from build123d import *

# Parameters (mm, degrees)
F1_DEPTH = 9.525
F2_DEPTH = 9.525
F3_D     = 12.7


with BuildPart() as f1:
    # F0 (on Right) → F1 (new body)
    with BuildSketch(Plane.YZ):
        Polygon((0, 57.15), (0, 0), (225.425, 0), (225.425, 37.3376765309), (225.425, 57.15), (156.083, 57.15), align=None)
    extrude(amount=F1_DEPTH)

    # F0 (on Right) → F2 (join)
    with BuildSketch(Plane.YZ):
        Polygon((0, 57.15), (0, 0), (225.425, 0), (225.425, 37.3376765309), (225.425, 57.15), (156.083, 57.15), align=None)
        with BuildLine():
            Line((225.425, 57.15), (225.425, 37.3376765309))
            Line((225.425, 37.3376765309), (319.5570650431, 64.2329913682))
            ThreePointArc((319.5570650431, 64.2329913682), (305.0721225399, 65.8972639905), (296.0065399278, 77.3164835165))
            Line((296.0065399278, 77.3164835165), (225.425, 57.15))
        make_face()
        with BuildLine():
            Line((309.0900320761, 100.8670086318), (156.083, 57.15))
            Line((156.083, 57.15), (225.425, 57.15))
            Line((225.425, 57.15), (296.0065399278, 77.3164835165))
            ThreePointArc((296.0065399278, 77.3164835165), (297.67081255, 91.8014260196), (309.0900320761, 100.8670086318))
        make_face()
        with BuildLine():
            Line((314.3235485596, 82.55), (319.5570650431, 64.2329913682))
            ThreePointArc((319.5570650431, 64.2329913682), (329.5321150438, 71.0782082701), (333.3735485596, 82.55))
            ThreePointArc((333.3735485596, 82.55), (325.7953402895, 97.7585664842), (309.0900320761, 100.8670086318))
            Line((309.0900320761, 100.8670086318), (314.3235485596, 82.55))
        make_face()
        with BuildLine():
            ThreePointArc((296.0065399278, 77.3164835165), (305.0721225399, 65.8972639905), (319.5570650431, 64.2329913682))
            Line((319.5570650431, 64.2329913682), (314.3235485596, 82.55))
            Line((314.3235485596, 82.55), (296.0065399278, 77.3164835165))
        make_face()
        with BuildLine():
            Line((314.3235485596, 82.55), (309.0900320761, 100.8670086318))
            ThreePointArc((309.0900320761, 100.8670086318), (297.67081255, 91.8014260196), (296.0065399278, 77.3164835165))
            Line((296.0065399278, 77.3164835165), (314.3235485596, 82.55))
        make_face()
    extrude(amount=F2_DEPTH)

    # F3 (through all)
    with Locations(Plane(origin=(0, 0, 0), x_dir=(0, 1, 0), z_dir=(-1, 0, 0))):
        with Locations((314.3235485596, -82.55)):
            Hole(F3_D / 2)


solid = f1.part
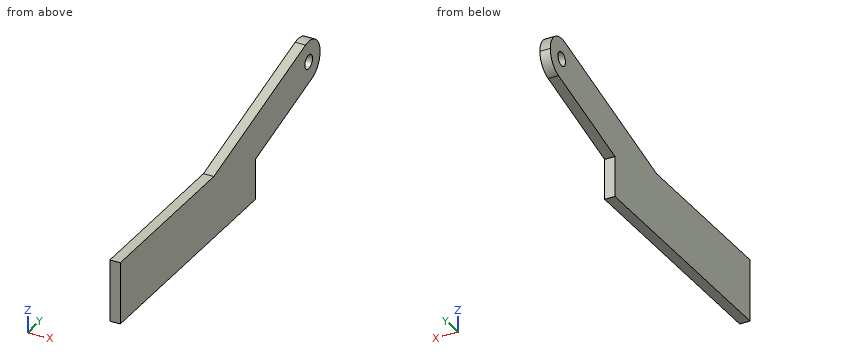
Part model, mm, in its own coordinate system. Give positions to 0.01 mm unless a question says otherwise; leave off trailing zeros. Loops run counter-clockwise (first coordinate to the right, second up) from the corner with the lowest first, then second, coordinate; pieces in that order, holes last. Notation, with made-up numbers: M 3.25,31 L 43.25,31 A30 cw 43.25,60 Z; hole C -10,8.25 d3. An arc over 180 degrees is marked long. Put each result on its own line as item: value. Start each with the question number.
1) Saw through at A-A (x = 6.5). List the corners of the cut face in (y, z) (3 decimals), then the cut area to 3 significant figures.
2) Saw through at C-C (y = 265.5). List the corners of the cut face in (x, z) (3 decimals), then the cut area to 3 significant figures.
3) Flat gauge pins, fed straight in: pin 1 (3 mm diameter, centred on x = 4, y = 82, fed in from +Z); pin 2 (5 mm diameter, centred on x = 7, z = 18, fed in from +Y) (3 decimals); pin 3 (4 mm diameter, centred on x = 7, y = 292, fed in from +Z); pin 4 (11.5 mm diameter, centred on y = 314.32, z = 82.55, fed in from +X). Where does each tip first touch, or does it go through?
4) Probe probe 1 along Z at (x, y) = (3, 150.5); probe 2 along Y at (x, z) = (3.5, 25) (3 decimals); probe 3 along Z at (x, y) = (4, 282). List the from-to ranges inside material, lowest first.
5) Saw through at B-B (y = 128). List the corners of the cut face in (x, z) (3 decimals).
Numbers:
1. outline: M 0,0 L 225.425,0 L 225.425,37.338 L 319.557,64.233 A19.05 ccw 309.09,100.867 L 156.083,57.15 L 0,57.15 Z; hole C 314.324,82.55 d12.7
1. area: 17,500 mm^2
2. outline: M 0,48.788 L 9.525,48.788 L 9.525,88.413 L 0,88.413 Z
2. area: 377 mm^2
3. pin 1: z = 57.15
3. pin 2: y = 225.425
3. pin 3: z = 96.56
3. pin 4: through
4. probe 1: 0 to 57.15
4. probe 2: 0 to 225.425
4. probe 3: 53.5 to 93.13
5. outline: M 0,0 L 9.525,0 L 9.525,57.15 L 0,57.15 Z
